Autodesk Inventor part; units mm, degrees
ref_plane "YZ Plane" through (0, 0, 0) normal (1, 0, 0) x (0, 1, 0)
ref_plane "XZ Plane" through (0, 0, 0) normal (0, 1, 0) x (-1, 0, 0)
ref_plane "XY Plane" through (0, 0, 0) normal (0, 0, 1) x (1, 0, 0)
sketch "Sketch1" plane through (0, 0, 0) normal (1, 0, 0) x (0, 1, 0)
  line L0 (0, 0) -> (914.4, 0)
  line L1 (914.4, 0) -> (914.4, -1625.6)
  line L2 (914.4, -1625.6) -> (0, -1625.6)
  line L3 (0, -1625.6) -> (0, 0)
  dimension "d0" = 1625.6
  dimension "d1" = 914.4
extrude "Extrusion1" add sketch "Sketch1" along normal blind 12.7
sketch "Sketch3" plane through (12.7, 0, 0) normal (1, 0, 0) x (0, 0, -1)
  line L0 (0, 0) -> (1625.6, 0)
  line L1 (1625.6, 0) -> (1625.6, 914.4)
  line L2 (127, 838.2) -> (1016, 838.2)
  line L3 (1016, 838.2) -> (1016, 635)
  line L4 (1016, 635) -> (127, 635)
  line L5 (127, 635) -> (127, 838.2)
  line L6 (0, 914.4) -> (0, 0)
  line L7 (1092.2, 838.2) -> (1498.6, 838.2)
  line L8 (1498.6, 838.2) -> (1498.6, 431.8)
  line L9 (1498.6, 431.8) -> (1092.2, 431.8)
  line L10 (1092.2, 431.8) -> (1092.2, 838.2)
  line L11 (1625.6, 914.4) -> (0, 914.4)
  dimension "d12" = 889
  dimension "d13" = 203.2
  dimension "d14" = 127
  dimension "d15" = 406.4
  dimension "d16" = 406.4
  dimension "d17" = 76.2
  dimension "d18" = 76.2
  dimension "d19" = 127
extrude "Extrusion3" cut sketch "Sketch3" against normal blind 127 contours L2 L3 L4 L5 | L7 L8 L9 L10
properties part number "HPStationBase-ver1-1111-2021" material "Aluminum 6061"
Model file for the job. Use its own axes, mm. Coordinates: 2 decimals unless noted, no trailing zeros. Write each loop counter-clockwise with the first axis right and the second up, starting at its lowest first coordinate (ties: lowest second). Pieces come first, ordered by that corner, then holes. Notation, with made-up numbers: (59, 58) -> (87, 58) arc R6 cw to (87, 68) -> close; hole circle Ø4 at (-38.5, 73.5). An arc over 180 degrees is marked (long way). One line per item, written item: value. Start each with the question number.
1) Slice it at B-B on z = -1292. Write the cut outline in (x, y).
2) Slice it at D-D on x = 2.25. Write the cut outline in (y, z), then the cut area to 3 significant figures.
3) Slice it at A-A on y = 721. Write the cut outline in (x, z), then the cut area to 3 significant figures.
4) Probe probe 1 along Z at (x, y) = (10, 727.5); probe 2 along Y at (x, z) = (7.25, -1374.5); probe 3 along Z at (x, y) = (5.5, 448). List the from-to ranges inside material, lowest first.
5) Slice it at C-C on y = 447. Write the cut outline in (x, z), then the cut area to 3 significant figures.
Answers follow:
1. outline: (0, 0) -> (12.7, 0) -> (12.7, 431.8) -> (0, 431.8) -> close; (0, 838.2) -> (12.7, 838.2) -> (12.7, 914.4) -> (0, 914.4) -> close
2. outline: (0, -1625.6) -> (914.4, -1625.6) -> (914.4, 0) -> (0, 0) -> close; hole (431.8, -1498.6) -> (838.2, -1498.6) -> (838.2, -1092.2) -> (431.8, -1092.2) -> close; hole (635, -1016) -> (838.2, -1016) -> (838.2, -127) -> (635, -127) -> close
2. area: 1,140,000 mm2
3. outline: (0, -1625.6) -> (12.7, -1625.6) -> (12.7, -1498.6) -> (0, -1498.6) -> close; (0, -1092.2) -> (12.7, -1092.2) -> (12.7, -1016) -> (0, -1016) -> close; (0, -127) -> (12.7, -127) -> (12.7, 0) -> (0, 0) -> close
3. area: 4,190 mm2
4. probe 1: -1625.6 to -1498.6, -1092.2 to -1016, -127 to 0
4. probe 2: 0 to 431.8, 838.2 to 914.4
4. probe 3: -1625.6 to -1498.6, -1092.2 to 0
5. outline: (0, -1625.6) -> (12.7, -1625.6) -> (12.7, -1498.6) -> (0, -1498.6) -> close; (0, -1092.2) -> (12.7, -1092.2) -> (12.7, 0) -> (0, 0) -> close
5. area: 15,500 mm2
